The listing builds one solid part. Answer for the finished solid, in the listing's coordinates (mm). Face numbers are marked on the shaded views. A direction names the side the tool comes from. Coordinates: 2 decimals unless noted, no trailing zeros. Loops run counter-clockwise (first coordinate to the right, second up) from the corner with the lowest first, then second, coordinate; pieces in that order, holes last. Notation, with made-up numbers: M 1,56.5 L 27,56.5 A19 cw 27,66.5 Z; hole C -15.5,51.25 d10. An arc over 180 degrees is marked long. Answer as a JSON object with one key per item and string values. Group by question number.
1. For the marked faces 4, 5 and 6, determine the directions among +Z, -Z, +X, -X, +Y, -Y from which every point of the face is accessible in a straight line to the end or side of a thin tool.
2. A cutting plane is placed at B-B on x = 15. Give the vertices of the cut face in (y, z).
3. Given pin 1 (12 mm diameter, centred on x = 31, y = 40, fed in from +Z); pin 2 (10 mm diameter, centred on y = 48.5, z = 13.5, fed in from +X); pin 3 (12.5 mm diameter, centred on x = -16, z = 15, fed in from +Y); pin 4 (3 mm diameter, centred on x = -15.5, y = 37.5, fed in from +Z), each flat-ended and moving along its own axis, determine where each tip first touches the part or whether it passes through.
4. Straight lines are drawn through the part: L1, parallel to Y at x = 3, z = 10.25; L2, parallel to X at y = 70, z = 11; L3, parallel to Y at x = 35, z = 7.5. For each, find the intervals that lie inside material, in ascending order.
5. A cutting plane is placed at C-C on y = 57. Give the vertices of the cut face in (x, z).
6. A cutting plane is placed at A-A on z = 15. Give the vertices of the cut face in (x, y), and give its area (3 significant figures).
7. Determine the mould class of the marked faces 1, 2 and 3 for opening direction Y: released by +Y, released by -Y, zero draft, split by the parting line, or undercut.
from build123d import *

# Parameters (mm, degrees)
F1_DEPTH = 25.4
F2_T     = -2.54


with BuildPart() as f1:
    # F0 (on Top) → F1 (new body)
    with BuildSketch(Plane.XY):
        Polygon((0, 130.1105469465), (0, 79.9251422286), (23.2478752732, 79.9251422286), (46.4957505465, 79.9251422286), (46.4957505465, 130.1105469465), align=None)
        Polygon((23.2478752732, 79.9251422286), (0, 79.9251422286), (-30.9502854943, 79.9251422286), (-30.9502854943, 0), (23.2478752732, 0), align=None)
    extrude(amount=F1_DEPTH)

    # F2
    f2_openings = [f1.faces().sort_by_distance(p)[0] for p in [
        (5.635859, 62.737644, 25.4),
    ]]
    offset(amount=F2_T, openings=f2_openings, kind=Kind.INTERSECTION)


solid = f1.part
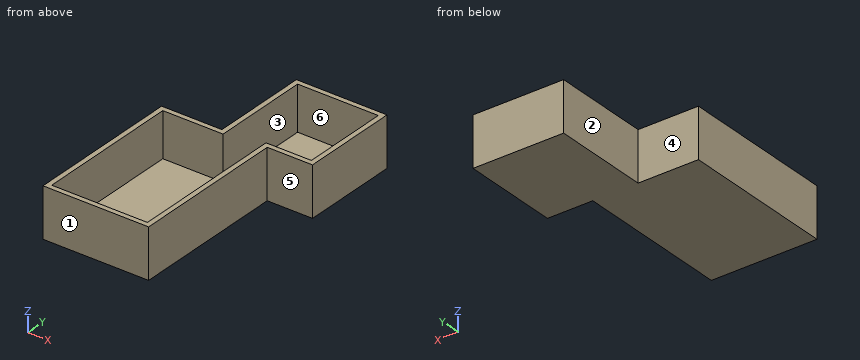
From the geometry:
{
 "1": {"face 4": "+Z, -Z, -X, +Y", "face 5": "+Z, -Z, +X, -Y", "face 6": "+Z"},
 "2": {"outline": "M 0,0 L 130.11,0 L 130.11,25.4 L 127.57,25.4 L 127.57,2.54 L 2.54,2.54 L 2.54,25.4 L 0,25.4 Z"},
 "3": {"pin 1": "passes through", "pin 2": "stops at x = 23.25", "pin 3": "stops at y = 79.93", "pin 4": "stops at z = 2.54"},
 "4": {"L1": "y = 0 to 2.54, 127.57 to 130.11", "L2": "x = -30.95 to -28.41, 20.71 to 23.25", "L3": "y = 79.93 to 82.47, 127.57 to 130.11"},
 "5": {"outline": "M -30.95,0 L 23.25,0 L 23.25,25.4 L 20.71,25.4 L 20.71,2.54 L -28.41,2.54 L -28.41,25.4 L -30.95,25.4 Z"},
 "6": {"outline": "M -30.95,0 L 23.25,0 L 23.25,79.93 L 46.5,79.93 L 46.5,130.11 L 0,130.11 L 0,79.93 L -30.95,79.93 Z; hole M -28.41,2.54 L 20.71,2.54 L 20.71,82.47 L 43.96,82.47 L 43.96,127.57 L 2.54,127.57 L 2.54,77.39 L -28.41,77.39 Z", "area": "1,030 mm²"},
 "7": {"face 1": "released by -Y", "face 2": "zero draft", "face 3": "undercut"}
}
